Input: dimensioned drawing with shaded views. Units: mm. Origin: part minimum x, y, z. A direction names the side the tool comes from. Give positions to 0.01 mm unless a question says otherwise; leave off trailing zeros. Write each loop counter-clockwise with the first axis right and the second up, starting at its lowest first coordinate (ties: lowest second). Pieces come first, ordered by that corner, then holes.
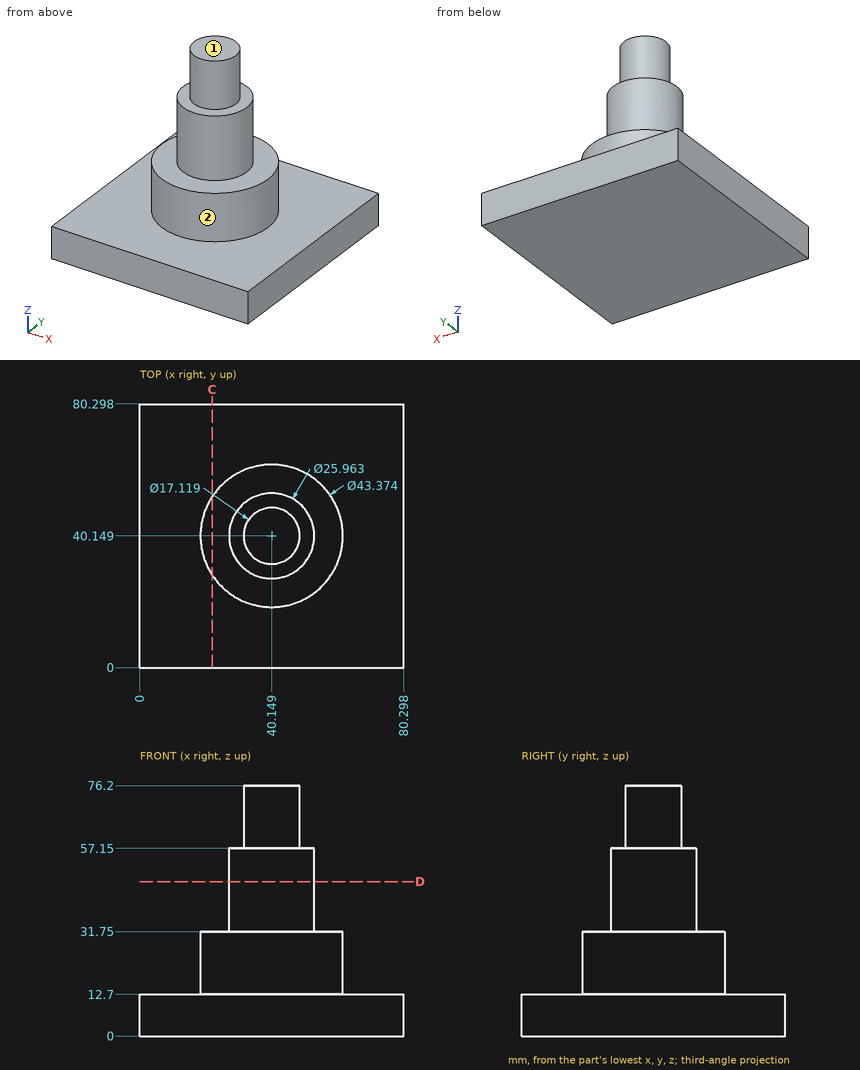
Item 1: Section C-C, the plane x = 22. Return the cut outline in (y, z), plus the area to 3 significant figures.
Found:
outline: (0, 0) - (80.3, 0) - (80.3, 12.7) - (52.02, 12.7) - (52.02, 31.75) - (28.28, 31.75) - (28.28, 12.7) - (0, 12.7) - close
area: 1,470 mm2
Item 2: Reachability of the marked faces 1 and 2 from +Z, -Z, +X, -X, +Y, -Y: full face, straight path, thin tool, end or side. Return the list, or none.
Found:
face 1: +Z, +X, -X, +Y, -Y
face 2: +Z
Item 3: Line query: L1, parallel to Z at x = 34.5, y = 48.5; L2, parallel to Z at x = 65, y = 68.5; L3, parallel to X at y = 39.5, z = 62. Output: solid intervals per line, ascending.
Found:
L1: z = 0 to 57.15
L2: z = 0 to 12.7
L3: x = 31.61 to 48.68
Item 4: Section D-D, the plane z = 47. Return the cut outline in (x, y), plus the area to 3 significant figures.
Found:
outline: circle Ø25.96 at (40.15, 40.15)
area: 529 mm2
Item 5: Pin query (flat end, axial travel): pin 1 Ø6 at (x, y) = (71.5, 17) entering from +Z; pin 2 Ø3 at (y, z) = (36.5, 32) entering from -X; pin 3 Ø8 at (y, z) = (56, 35) entering from +X. Return the tip coordinate at first contact, or that it passes through.
Found:
pin 1: stops at z = 12.7
pin 2: stops at x = 18.57
pin 3: stops at x = 57.11
